Work out the finished part from the listing and answer in its coordinate system (mm). Face numbers are marked on the shaded views. A direction names the side the tool comes from. Round coordinates to 2 decimals unless told otherwise and drop trailing zeros. Loops run counter-clockwise (first coordinate to the right, second up) from the corner with the lowest first, then second, coordinate; pieces in that order, holes last. Notation, with made-up numbers: (17.5, -14.5) -> (40.5, -14.5) arc R22 ccw to (40.5, 0.5) -> close; hole circle Ø6 at (50, 55). An arc over 180 degrees is marked (long way). Use CSV: the item, a comma, the result in double quotes. Start each with the question number.
from build123d import *

# Parameters (mm, degrees)
F0_W      = 40
F0_H      = 40
F1_DEPTH  = 80
F2_W      = 10
F2_H      = 40
F3_DEPTH  = 40
F4_R      = 19.99999
F5_R      = 5
F6_DEPTH  = 40.001
F7_R      = 5
F8_DEPTH  = 30
F9_W      = 40
F9_H      = 40
F10_DEPTH = 50
F12_DEPTH = 50.001


# Not quite as in the source:
# - a fillet or chamfer is up to 0.001 mm smaller than in the source, because OpenCascade refuses the exact size


with BuildPart() as f1:
    # F0 (on Right) → F1 (new body)
    with BuildSketch(Plane.YZ):
        Rectangle(F0_W, F0_H)
    extrude(amount=F1_DEPTH)

    # F2 (on face) → F3 (join)
    with BuildSketch(Plane(origin=(0, 0, 0), x_dir=(0, -1, 0), z_dir=(-1, 0, 0))):
        with Locations((15, 0)):
            Rectangle(F2_W, F2_H)
        with Locations((-15, 0)):
            Rectangle(F2_W, F2_H)
    extrude(amount=F3_DEPTH)

    # F4 (radius 20 in the source; OpenCascade refuses exactly that, so slightly less here)
    f4_edges = [f1.edges().sort_by_distance(p)[0] for p in [
        (-40, 15, 20),
        (-40, 15, -20),
        (-40, -15, 20),
        (-40, -15, -20),
    ]]
    fillet(f4_edges, radius=F4_R)

    # F5 (on face) → F6 (cut, through all)
    with BuildSketch(Plane.XZ.offset(20)):
        with Locations((-20, 0)):
            Circle(F5_R)
    extrude(amount=-F6_DEPTH, mode=Mode.SUBTRACT)

    # F7 (on Front) → F8 (join, symmetric)
    with BuildSketch(Plane.XZ):
        with Locations((40, 0)):
            Circle(F7_R)
    extrude(amount=F8_DEPTH, both=True)

    # F9 (on face) → F10 (join)
    with BuildSketch(Plane.YZ.offset(80)):
        Rectangle(F9_W, F9_H)
    extrude(amount=F10_DEPTH)

    # F11 (on face) → F12 (cut, through all)
    with BuildSketch(Plane.XZ.offset(20)):
        Polygon((60, 20), (130, 0), (130, 20), align=None)
        Polygon((130, -20), (130, -10), (60, -20), align=None)
    extrude(amount=-F12_DEPTH, mode=Mode.SUBTRACT)


solid = f1.part
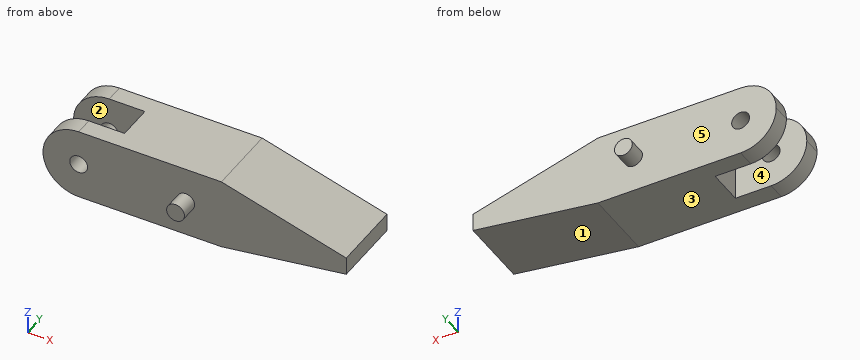
Q1. Section D-D, the plane y = -0.5 is taken. Write down the section's boundary in (x, z).
Q2. Section C-C, the plane z = 14.5 is taken. Write down the section's boundary in (x, y), and give its area (3 significant figures).
Q3. For a pull along Y with two mould halves and no side action, classify the marked faces 3, 4 and 5 as pulls with the +Y half, pulls with the -Y half, needs draft (parallel to the pull), parting line crosses it, or undercut.
Q4. Which of the six approach directions +Z, -Z, +X, -X, +Y, -Y give full straight-line access (tool end or side, diameter ignored) to the marked faces 1 and 2?
Q5. Each of these flat-tipped pins is pushed along its axis until it touches: pin 1 (12 mm diameter, centred on x = -13, z = -9, fed in from -Y); pin 2 (20 mm diameter, centred on x = 3, z = 0, fed in from +Y). Where does it stop, or does it pass through?
Q6. Section B-B, the plane x = 40 is taken. Write down the section's boundary in (y, z).
Q7. Straight lines are drawn through the part: line 1 (Y direction, x = -5.5, z = 17); line 2 (Z direction, x = -20, y = 15.5); line 3 (Y direction, x = 40.5, z = -6.5). For each, find the intervals that lie inside material, in ascending order. Write a range as from..to.
Report:
1,outline,"(0, -20) -> (60, -20) -> (130, -10) -> (130, 0) -> (60, 20) -> (0, 20) -> close"
2,outline,"(-33.77, -20) -> (79.25, -20) -> (79.25, 20) -> (-33.77, 20) -> (-33.77, 10) -> (0, 10) -> (0, -10) -> (-33.77, -10) -> close"
2,area,"3,850 mm²"
3,face 3,"needs draft"
3,face 4,"undercut"
3,face 5,"pulls with the +Y half"
4,face 1,"-Z, +X, +Y, -Y"
4,face 2,"+Z, -Z, -X"
5,pin 1,"stops at y = -20"
5,pin 2,"stops at y = 20"
6,outline,"(-30, -5) -> (-20, -5) -> (-20, -20) -> (20, -20) -> (20, -5) -> (30, -5) -> (30, 5) -> (20, 5) -> (20, 20) -> (-20, 20) -> (-20, 5) -> (-30, 5) -> close"
7,line 1,"y = -20..-10, 10..20"
7,line 2,"z = -20..-5, 5..20"
7,line 3,"y = -20..20"
